```python
from build123d import *

# Parameters (mm, degrees)
F1_DEPTH = 3.175


with BuildPart() as f1:
    # F0 (on Front) → F1 (new body)
    with BuildSketch(Plane.XZ):
        with BuildLine():
            Line((-4.7625, -49.2125), (19.05, -49.2125))
            Line((19.05, -49.2125), (19.05, 49.2125))
            Line((19.05, 49.2125), (-4.7625, 49.2125))
            ThreePointArc((-4.7625, 49.2125), (-14.865288, 45.027788), (-19.05, 34.925))
            Line((-19.05, 34.925), (-19.05, -34.925))
            ThreePointArc((-19.05, -34.925), (-14.865288, -45.027788), (-4.7625, -49.2125))
        make_face()
        with BuildLine():
            ThreePointArc((11.1125, -38.1), (9.252628, -42.590128), (4.7625, -44.45))
            Line((4.7625, -44.45), (-7.9375, -44.45))
            ThreePointArc((-7.9375, -44.45), (-12.427628, -42.590128), (-14.2875, -38.1))
            ThreePointArc((-14.2875, -38.1), (-12.427628, -33.609872), (-7.9375, -31.75))
            Line((-7.9375, -31.75), (4.7625, -31.75))
            ThreePointArc((4.7625, -31.75), (9.252628, -33.609872), (11.1125, -38.1))
        make_face(mode=Mode.SUBTRACT)
        with BuildLine():
            Line((-7.9375, -6.35), (4.7625, -6.35))
            ThreePointArc((4.7625, -6.35), (9.252628, -8.209872), (11.1125, -12.7))
            ThreePointArc((11.1125, -12.7), (9.252628, -17.190128), (4.7625, -19.05))
            Line((4.7625, -19.05), (-7.9375, -19.05))
            ThreePointArc((-7.9375, -19.05), (-12.427628, -17.190128), (-14.2875, -12.7))
            ThreePointArc((-14.2875, -12.7), (-12.427628, -8.209872), (-7.9375, -6.35))
        make_face(mode=Mode.SUBTRACT)
        with BuildLine():
            Line((-7.9375, 19.05), (4.7625, 19.05))
            ThreePointArc((4.7625, 19.05), (9.252628, 17.190128), (11.1125, 12.7))
            ThreePointArc((11.1125, 12.7), (9.252628, 8.209872), (4.7625, 6.35))
            Line((4.7625, 6.35), (-7.9375, 6.35))
            ThreePointArc((-7.9375, 6.35), (-12.427628, 8.209872), (-14.2875, 12.7))
            ThreePointArc((-14.2875, 12.7), (-12.427628, 17.190128), (-7.9375, 19.05))
        make_face(mode=Mode.SUBTRACT)
        with BuildLine():
            Line((-7.9375, 44.45), (4.7625, 44.45))
            ThreePointArc((4.7625, 44.45), (9.252628, 42.590128), (11.1125, 38.1))
            ThreePointArc((11.1125, 38.1), (9.252628, 33.609872), (4.7625, 31.75))
            Line((4.7625, 31.75), (-7.9375, 31.75))
            ThreePointArc((-7.9375, 31.75), (-12.427628, 33.609872), (-14.2875, 38.1))
            ThreePointArc((-14.2875, 38.1), (-12.427628, 42.590128), (-7.9375, 44.45))
        make_face(mode=Mode.SUBTRACT)
    extrude(amount=F1_DEPTH)


solid = f1.part
```
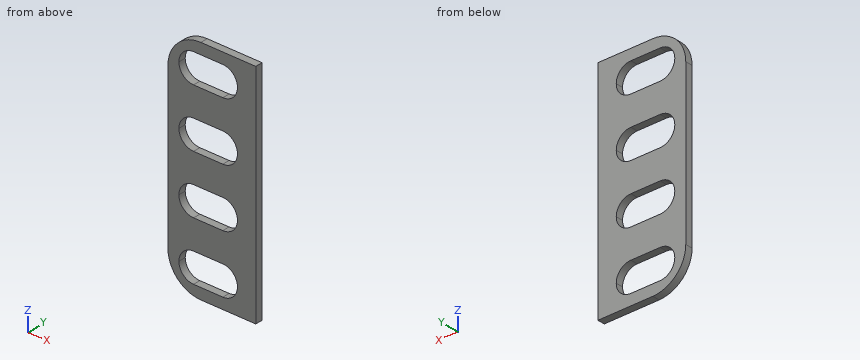
The listing builds one solid part. Answer for the finished solid, in the listing's coordinates (mm). Give positions to 0.01 mm unless a question says otherwise; leave off trailing zeros. Loops run counter-clockwise (first coordinate to the right, second up) from the corner with the lowest first, then second, coordinate; pieces in that order, holes last. Notation, with made-up numbers: M 75,51 L 104,51 A22 cw 104,75 Z; hole C -38,28.25 d10. An arc over 180 degrees is marked long. One line per item, written item: value.
Q1. A cutting plane is placed at A-A on x = -1.5. Give the number of separate pieces and of enclosed holes in the cut face, then the cut area to 3 significant figures.
Working result:
separate pieces: 5
enclosed holes: 0
area: 151 mm^2
Q2. Find the intervals of material crossed by line 1 (Z direction, x = -4, y = -0.15); line 2 (Z direction, x = -11.5, y = -1.5); line 3 (X direction, y = -0.2, z = -13.5), in increasing order. Write a range as from..to.
Working result:
line 1: z = -49.21..-44.45, -31.75..-19.05, -6.35..6.35, 19.05..31.75, 44.45..49.21
line 2: z = -47.52..-43.36, -32.84..-17.96, -7.44..7.44, 17.96..32.84, 43.36..47.52
line 3: x = -19.05..-14.24, 11.06..19.05
Q3. A cutting plane is placed at B-B on z = -43. Determine the outline of the cut face in (x, y) (3 decimals), then the cut area to 3 significant figures.
Working result:
outline: M -16.549,-3.175 L -11.976,-3.175 L -11.976,0 L -16.549,0 Z; M 8.801,-3.175 L 19.05,-3.175 L 19.05,0 L 8.801,0 Z
area: 47.1 mm^2
Q4. A cutting plane is placed at D-D on z = 9.5. Determine the outline of the cut face in (x, y) (3 decimals), then the cut area to 3 significant figures.
Working result:
outline: M -19.05,-3.175 L -13.422,-3.175 L -13.422,0 L -19.05,0 Z; M 10.247,-3.175 L 19.05,-3.175 L 19.05,0 L 10.247,0 Z
area: 45.8 mm^2
